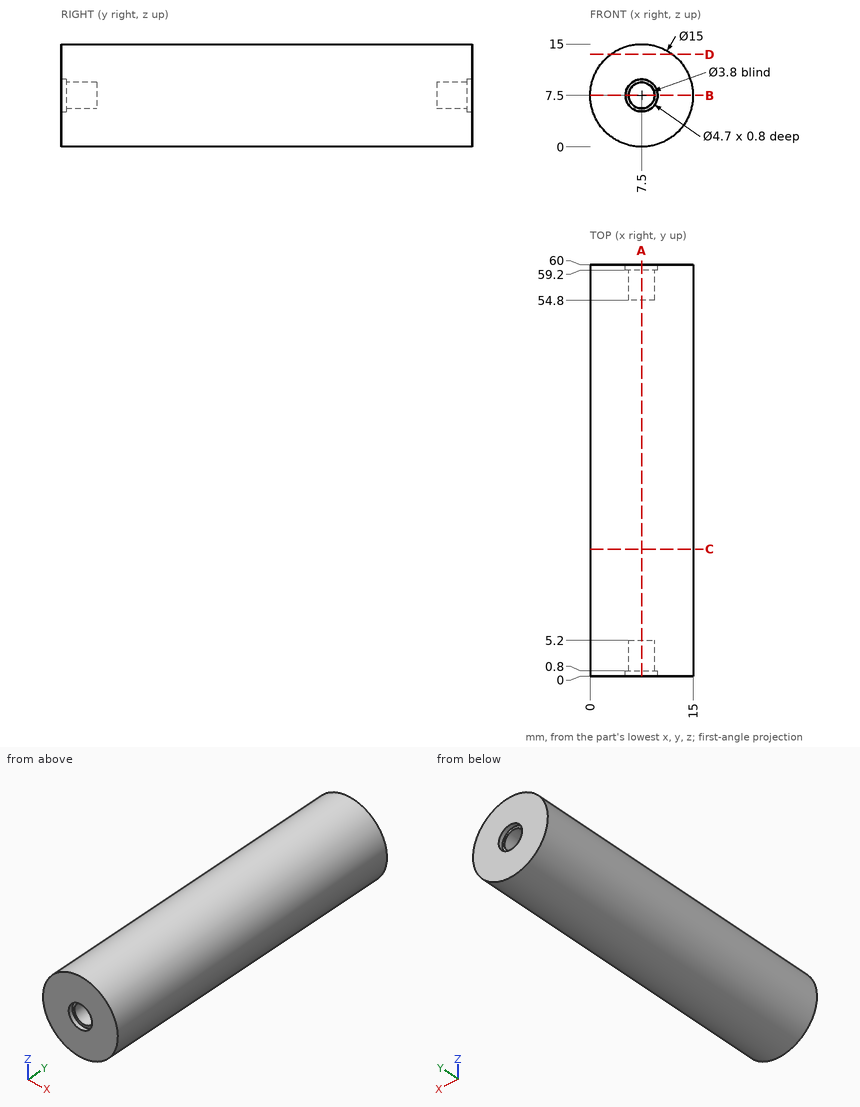
For this review, use the dimensioned drawing (mm, ordinates from the lowest corner) and the shaded views. Coordinates: 2 decimals unless noted, no trailing zeros. Order: outer loops, then holes, each group sorted by start corner. A loop starts at its lowest first (then second) coordinate and runs counter-clockwise, first axis right, second up. Notation, with made-up numbers: M -10,8 L 5,8 A14 ccw 5,17 Z; hole C 73.25,63 d10. An arc over 180 degrees is marked long. Answer as a JSON object with one key per item and string values. Group by question number.
1) Add section D-D, the plane z = 13.5. Write out the cut boundary in (x, y), then the cut area to 3 significant figures.
2) For pin 1 (4 mm diameter, centred on x = 2.5, y = 48.5, fed in from -Z); pin 2 (2.5 mm diameter, centred on x = 7.5, z = 7.5, fed in from -Y); pin 3 (1.5 mm diameter, centred on x = 6.5, y = 36, fed in from +Z), all flat-tipped, find the tip position at first contact; note any pin that passes through.
3) Add section A-A, the plane x = 7.5. Write out the cut boundary in (y, z).
4) Add section B-B, the plane z = 7.5. Write out the cut boundary in (x, y).
5) Add section C-C, the plane y = 18.5. Write out the cut boundary in (x, z).
6) Wall thickness on L1, parallel to X at y = 58.3, z = 7.5; L2, parallel to X at y = 59.8, z = 7.5; L3, parallel to X at y = 50, z = 13: over which ranges is each line inside the solid? List them lowest first.
Computed values:
{
 "1": {"outline": "M 3,0 L 12,0 L 12,60 L 3,60 Z", "area": "540 mm^2"},
 "2": {"pin 1": "stops at z = 0.63", "pin 2": "stops at y = 5.2", "pin 3": "stops at z = 15"},
 "3": {"outline": "M 0,0 L 60,0 L 60,5.15 L 59.2,5.15 L 59.2,5.6 L 54.8,5.6 L 54.8,9.4 L 59.2,9.4 L 59.2,9.85 L 60,9.85 L 60,15 L 0,15 L 0,9.85 L 0.8,9.85 L 0.8,9.4 L 5.2,9.4 L 5.2,5.6 L 0.8,5.6 L 0.8,5.15 L 0,5.15 Z"},
 "4": {"outline": "M 0,0 L 5.15,0 L 5.15,0.8 L 5.6,0.8 L 5.6,5.2 L 9.4,5.2 L 9.4,0.8 L 9.85,0.8 L 9.85,0 L 15,0 L 15,60 L 9.85,60 L 9.85,59.2 L 9.4,59.2 L 9.4,54.8 L 5.6,54.8 L 5.6,59.2 L 5.15,59.2 L 5.15,60 L 0,60 Z"},
 "5": {"outline": "C 7.5,7.5 d15"},
 "6": {"L1": "x = 0 to 5.6, 9.4 to 15", "L2": "x = 0 to 5.15, 9.85 to 15", "L3": "x = 2.4 to 12.6"}
}
